Design review of the part built by this model. Coordinates are the model's own, in mm. A direction names the side the tool comes from. Round coordinates to 2 decimals unless told otherwise and drop trailing zeros. Order: outer loops, then holes, each group sorted by start corner. A loop starts at its lowest first (then second) coordinate and runs counter-clockwise, first axis right, second up. Notation, with made-up numbers: (53.5, 65) - (68.5, 65) arc R36 cw to (68.5, 101) - close; hole circle Ø8 at (68, 51). An arc over 180 degrees is marked (long way). Write item = value, one per line.
from build123d import *

# Parameters (mm, degrees)
SKETCH1_W           = 60
SKETCH1_H           = 60
BOSS_EXTRUDE1_DEPTH = 56
FILLET1_R           = 4
SHELL1_T            = -1.6
CUT_EXTRUDE1_DEPTH  = 69.988114918
BOSS_EXTRUDE2_START = 8
BOSS_EXTRUDE2_DEPTH = 8
CUT_EXTRUDE2_REACH  = 78.245
SKETCH3_R           = 2.4
CUT_EXTRUDE3_REACH  = 89.384


with BuildPart() as part:
    # Sketch1 → Boss-Extrude1 (new body)
    with BuildSketch(Plane(origin=(0, 0, 0), x_dir=(1, 0, 0), z_dir=(0, 1, 0))):
        Rectangle(SKETCH1_W, SKETCH1_H)
    extrude(amount=BOSS_EXTRUDE1_DEPTH)

    # Fillet1
    fillet1_edges = [part.edges().sort_by_distance(p)[0] for p in [
        (0, 0, 30),
        (-30, 0, 0),
        (0, 0, -30),
        (30, 0, 0),
        (30, 28, 30),
        (-30, 28, 30),
        (-30, 28, -30),
        (30, 28, -30),
    ]]
    fillet(fillet1_edges, radius=FILLET1_R)

    # Shell1
    shell1_openings = [part.faces().sort_by_distance(p)[0] for p in [
        (0, 56, 0),
    ]]
    offset(amount=SHELL1_T, openings=shell1_openings, kind=Kind.INTERSECTION)

    # Sketch2 → Cut-Extrude1 (cut, through all)
    with BuildSketch(Plane(origin=(0, 1.6, 0), x_dir=(1, 0, 0), z_dir=(0, 1, 0))):
        with BuildLine():
            Line((18.864939852, 1.60266636), (12.761084932, 8.2247849))
            ThreePointArc((12.761084932, 8.2247849), (10.757749844, 9.653700125), (8.349320226, 10.158295975))
            Line((8.349320226, 10.158295975), (-8.295911111, 10.158295975))
            ThreePointArc((-8.295911111, 10.158295975), (-10.704340729, 9.653700125), (-12.707675817, 8.2247849))
            Line((-12.707675817, 8.2247849), (-18.811530736, 1.60266636))
            ThreePointArc((-18.811530736, 1.60266636), (-19.473295442, -0.091704025), (-18.811530736, -1.786074411))
            Line((-18.811530736, -1.786074411), (-12.707675817, -8.408192951))
            ThreePointArc((-12.707675817, -8.408192951), (-10.704340729, -9.837108176), (-8.295911111, -10.341704025))
            Line((-8.295911111, -10.341704025), (8.349320226, -10.341704025))
            ThreePointArc((8.349320226, -10.341704025), (10.757749844, -9.837108176), (12.761084932, -8.408192951))
            Line((12.761084932, -8.408192951), (18.864939852, -1.786074411))
            ThreePointArc((18.864939852, -1.786074411), (19.526704558, -0.091704025), (18.864939852, 1.60266636))
        make_face()
    extrude(amount=-CUT_EXTRUDE1_DEPTH, mode=Mode.SUBTRACT)

    # Sketch2<4> → Boss-Extrude2 (add)
    with BuildSketch(Plane(origin=(0, 1.6, 0), x_dir=(1, 0, 0), z_dir=(0, 1, 0)).offset(BOSS_EXTRUDE2_START)):
        with BuildLine():
            Line((20.335528087, 2.958162669), (14.231673168, 9.580281209))
            ThreePointArc((14.231673168, 9.580281209), (11.560559717, 11.485501509), (8.349320226, 12.158295975))
            Line((8.349320226, 12.158295975), (-8.295911111, 12.158295975))
            ThreePointArc((-8.295911111, 12.158295975), (-11.507150601, 11.485501509), (-14.178264052, 9.580281209))
            Line((-14.178264052, 9.580281209), (-20.282118972, 2.958162669))
            ThreePointArc((-20.282118972, 2.958162669), (-21.473295442, -0.091704025), (-20.282118972, -3.141570719))
            Line((-20.282118972, -3.141570719), (-14.178264052, -9.763689259))
            ThreePointArc((-14.178264052, -9.763689259), (-11.507150601, -11.668909559), (-8.295911111, -12.341704025))
            Line((-8.295911111, -12.341704025), (8.349320226, -12.341704025))
            ThreePointArc((8.349320226, -12.341704025), (11.560559717, -11.668909559), (14.231673168, -9.763689259))
            Line((14.231673168, -9.763689259), (20.335528087, -3.141570719))
            ThreePointArc((20.335528087, -3.141570719), (21.526704558, -0.091704025), (20.335528087, 2.958162669))
        make_face()
        with BuildLine():
            Line((18.864939852, 1.60266636), (12.761084932, 8.2247849))
            ThreePointArc((12.761084932, 8.2247849), (10.757749844, 9.653700125), (8.349320226, 10.158295975))
            Line((8.349320226, 10.158295975), (-8.295911111, 10.158295975))
            ThreePointArc((-8.295911111, 10.158295975), (-10.704340729, 9.653700125), (-12.707675817, 8.2247849))
            Line((-12.707675817, 8.2247849), (-18.811530736, 1.60266636))
            ThreePointArc((-18.811530736, 1.60266636), (-19.473295442, -0.091704025), (-18.811530736, -1.786074411))
            Line((-18.811530736, -1.786074411), (-12.707675817, -8.408192951))
            ThreePointArc((-12.707675817, -8.408192951), (-10.704340729, -9.837108176), (-8.295911111, -10.341704025))
            Line((-8.295911111, -10.341704025), (8.349320226, -10.341704025))
            ThreePointArc((8.349320226, -10.341704025), (10.757749844, -9.837108176), (12.761084932, -8.408192951))
            Line((12.761084932, -8.408192951), (18.864939852, -1.786074411))
            ThreePointArc((18.864939852, -1.786074411), (19.526704558, -0.091704025), (18.864939852, 1.60266636))
        make_face(mode=Mode.SUBTRACT)
    extrude(amount=-BOSS_EXTRUDE2_DEPTH)

    # Cut-Extrude2: up to this face of the body (flat: up to its plane)
    cut_extrude2_end = Plane(part.part.faces().sort_by_distance((0.026704558, 5.6, 12.341704025))[0])
    # Sketch3 → Cut-Extrude2 (cut, up to the picked face)
    with BuildSketch(Plane(origin=(0, 0, -12.158295975), x_dir=(-1, 0, 0), z_dir=(0, 0, -1)), mode=Mode.PRIVATE) as cut_extrude2_sk1:
        with Locations((-0.026704558, 5.6)):
            Circle(SKETCH3_R)
    cut_extrude2_tool1 = split(extrude(cut_extrude2_sk1.sketch, amount=-CUT_EXTRUDE2_REACH, mode=Mode.PRIVATE), bisect_by=cut_extrude2_end, keep=Keep.BOTH, mode=Mode.PRIVATE)
    add(cut_extrude2_tool1.solids().sort_by(Axis((0.026705, 5.6, -12.158296), (0, 0, 1)))[0], mode=Mode.SUBTRACT)

    # Cut-Extrude3: up to this face of the body (flat: up to its plane)
    cut_extrude3_end = Plane(part.part.faces().sort_by_distance((-30, 30, 0))[0])
    # Sketch4 → Cut-Extrude3 (cut, up to the picked face)
    with BuildSketch(Plane(origin=(30, 0, 0), x_dir=(0, 0, -1), z_dir=(1, 0, 0)), mode=Mode.PRIVATE) as cut_extrude3_sk1:
        with BuildLine():
            ThreePointArc((2, 51), (1.414213562, 52.414213562), (0, 53))
            Line((0, 53), (0, 49))
            ThreePointArc((0, 49), (1.414213562, 49.585786438), (2, 51))
        make_face()
    cut_extrude3_tool1 = split(extrude(cut_extrude3_sk1.sketch, amount=-CUT_EXTRUDE3_REACH, mode=Mode.PRIVATE), bisect_by=cut_extrude3_end, keep=Keep.BOTH, mode=Mode.PRIVATE)
    # Sketch4 → Cut-Extrude3 (cut, up to the picked face)
    with BuildSketch(Plane(origin=(30, 0, 0), x_dir=(0, 0, -1), z_dir=(1, 0, 0)), mode=Mode.PRIVATE) as cut_extrude3_sk2:
        with BuildLine():
            Line((0, 49), (0, 53))
            ThreePointArc((0, 53), (-2, 51), (0, 49))
        make_face()
    cut_extrude3_tool2 = split(extrude(cut_extrude3_sk2.sketch, amount=-CUT_EXTRUDE3_REACH, mode=Mode.PRIVATE), bisect_by=cut_extrude3_end, keep=Keep.BOTH, mode=Mode.PRIVATE)
    # Sketch4 → Cut-Extrude3 (cut, up to the picked face)
    with BuildSketch(Plane(origin=(30, 0, 0), x_dir=(0, 0, -1), z_dir=(1, 0, 0)), mode=Mode.PRIVATE) as cut_extrude3_sk3:
        with BuildLine():
            ThreePointArc((2, 51), (1.414213562, 52.414213562), (0, 53))
            Line((0, 53), (0, 49))
            ThreePointArc((0, 49), (1.414213562, 49.585786438), (2, 51))
        make_face()
    cut_extrude3_tool3 = split(extrude(cut_extrude3_sk3.sketch, amount=-CUT_EXTRUDE3_REACH, mode=Mode.PRIVATE), bisect_by=cut_extrude3_end, keep=Keep.BOTH, mode=Mode.PRIVATE)
    # Sketch4 → Cut-Extrude3 (cut, up to the picked face)
    with BuildSketch(Plane(origin=(30, 0, 0), x_dir=(0, 0, -1), z_dir=(1, 0, 0)), mode=Mode.PRIVATE) as cut_extrude3_sk4:
        with BuildLine():
            Line((0, 49), (0, 53))
            ThreePointArc((0, 53), (-2, 51), (0, 49))
        make_face()
    cut_extrude3_tool4 = split(extrude(cut_extrude3_sk4.sketch, amount=-CUT_EXTRUDE3_REACH, mode=Mode.PRIVATE), bisect_by=cut_extrude3_end, keep=Keep.BOTH, mode=Mode.PRIVATE)
    add(cut_extrude3_tool1.solids().sort_by(Axis((30, 51, -0.848826), (-1, 0, 0)))[0], mode=Mode.SUBTRACT)
    add(cut_extrude3_tool2.solids().sort_by(Axis((30, 51, 0.848826), (-1, 0, 0)))[0], mode=Mode.SUBTRACT)
    add(cut_extrude3_tool3.solids().sort_by(Axis((30, 51, -0.848826), (-1, 0, 0)))[0], mode=Mode.SUBTRACT)
    add(cut_extrude3_tool4.solids().sort_by(Axis((30, 51, 0.848826), (-1, 0, 0)))[0], mode=Mode.SUBTRACT)


solid = part.part
Item 1: Take a section at D-D, the plane x = 11. State the section outline as (y, z) points, and give its area (3 significant figures).
Data:
outline = (0, -26) arc R4 ccw to (4, -30) - (56, -30) - (56, -28.4) - (4, -28.4) arc R2.4 cw to (1.6, -26) - (1.6, -11.71) - (9.6, -11.71) - (9.6, -9.54) - (0, -9.54) - close; (0, 9.72) - (9.6, 9.72) - (9.6, 11.89) - (1.6, 11.89) - (1.6, 26) arc R2.4 cw to (4, 28.4) - (56, 28.4) - (56, 30) - (4, 30) arc R4 ccw to (0, 26) - close
area = 270 mm2
Item 2: Insertion check: P1, Ø3, axis at x = -3.5, z = 14.5, coming from the +Y side. The pin has a flat end and moves straight along its axis. Give the tip position at first contact, or say it passes through.
Data:
P1 = 1.6
Item 3: Take a section at B-B, the plane z = 21.5. State the section outline as (x, y) points, and give its area (3 significant figures).
Data:
outline = (-30, 4) arc R4 ccw to (-26, 0) - (26, 0) arc R4 ccw to (30, 4) - (30, 56) - (28.4, 56) - (28.4, 4) arc R2.4 cw to (26, 1.6) - (-26, 1.6) arc R2.4 cw to (-28.4, 4) - (-28.4, 56) - (-30, 56) - close
area = 266 mm2
Item 4: Take a section at C-C, the plane x = -24.5. State the section outline as (y, z) points, and give its area (3 significant figures).
Data:
outline = (0, -26) arc R4 ccw to (4, -30) - (56, -30) - (56, -28.4) - (4, -28.4) arc R2.4 cw to (1.6, -26) - (1.6, 26) arc R2.4 cw to (4, 28.4) - (56, 28.4) - (56, 30) - (4, 30) arc R4 ccw to (0, 26) - close
area = 266 mm2
Item 5: The part is to be moulded in two halves that separate along Y. For faces 4 (the face through (0.547, 3.257, -11.172)), 5 (the face through (-12, 1.6, -12)), 6 (the face through (-28.859, 1.203, -0.364)), 7 (the face through (10.73, 4.87, 9.85)), say which applies: +Y half, -Y half, draft (parallel to the pull), parting line (faces both ways), or undercut.
Data:
face_4 = undercut
face_5 = +Y half
face_6 = -Y half
face_7 = draft
Item 6: For faces 1 (the face through (28.797, 30.364, 28.859)), 2 (the face through (15.856, 4.867, -4.867)), 3 (the face through (0, 30, 28.4)), list the 3-axis set-ups (+Z, -Z, +X, -X, +Y, -Y) from which the entire face can be reached by the end or side of a thin tool; tool diameter is ignored.
Data:
face_1 = +Z, +X, +Y, -Y
face_2 = +Y, -Y
face_3 = +Y
Item 7: Take a section at A-A, the plane y = 40.5. State the section outline as (x, z) points.
Data:
outline = (-30, -26) arc R4 ccw to (-26, -30) - (26, -30) arc R4 ccw to (30, -26) - (30, 26) arc R4 ccw to (26, 30) - (-26, 30) arc R4 ccw to (-30, 26) - close; hole (-28.4, -26) arc R2.4 ccw to (-26, -28.4) - (26, -28.4) arc R2.4 ccw to (28.4, -26) - (28.4, 26) arc R2.4 ccw to (26, 28.4) - (-26, 28.4) arc R2.4 ccw to (-28.4, 26) - close
Item 8: For line 1 along X through (y, z) = (33.5, 4); line 2 along Z through (x, y) = (-2.5, 5.5), list the stretches that pass through material, from the lowest coordinate up. Write a range as [from, to].
Data:
line_1 = [-30, -28.4], [28.4, 30]
line_2 = [-30, -28.4], [-12.16, -10.16], [10.34, 12.34], [28.4, 30]
